Design review of the part built by this model. Coordinates are the model's own, in mm. A direction names the side the tool comes from. Coordinates: 2 decimals unless noted, no trailing zeros. Write item = value, one per line.
```python
from build123d import *

# Parameters (mm, degrees)
F1_DEPTH    = 9
F2_T        = -1.625
F3_R        = 4.65
F4_DEPTH    = 5.75
F6_DEPTH    = 9
F7_T4_DEPTH = 11.5292765407
F8_R        = 1.5
F9_R        = 1.5
F11_DEPTH   = 25
F12_R       = 1.65
F13_DEPTH   = 0.8125
F14_R       = 4.65
F14_R_2     = 1.65
F15_DEPTH   = 0.8125
F17_DEPTH   = 25
F19_DEPTH   = 25


# Not quite as in the source:
# - a fillet or chamfer that OpenCascade refuses, or shapes differently, is made with other operations: its cross-section is extruded or revolved along the edge and cut away or added


with BuildPart() as f1:
    # F0 (on Top) → F1 (new body)
    with BuildSketch(Plane.XY):
        with BuildLine():
            Line((-2.2380131875, 10.0346875), (0, 9.35))
            Line((0, 9.35), (9.2696152423, -6.7054445662))
            Line((9.2696152423, -6.7054445662), (0, -6.7054445662))
            Line((0, -6.7054445662), (4.6188021535, -14.7054445662))
            Line((4.6188021535, -14.7054445662), (12.7337168574, -14.7054445662))
            ThreePointArc((12.7337168574, -14.7054445662), (17.9298692801, -11.7054445662), (17.9298692801, -5.7054445662))
            Line((17.9298692801, -5.7054445662), (14, 1.101288694))
            ThreePointArc((14, 1.101288694), (12.0019915499, 16.2776695961), (21.3205080757, 28.4217967697))
            Line((21.3205080757, 28.4217967697), (25.6506350946, 30.9217967697))
            ThreePointArc((25.6506350946, 30.9217967697), (29.1558482852, 35.7019755006), (28, 41.5158075373))
            Line((28, 41.5158075373), (-6.2733497352, 21.7280798417))
            ThreePointArc((-6.2733497352, 21.7280798417), (-7.2315061235, 14.8544401058), (-2.2380131875, 10.0346875))
        make_face()
        with BuildLine():
            ThreePointArc((1.65, 17.35), (1.166726189, 16.183273811), (0, 15.7))
            ThreePointArc((0, 15.7), (-1.166726189, 18.516726189), (1.65, 17.35))
        make_face(mode=Mode.SUBTRACT)
    extrude(amount=F1_DEPTH)

    # F2
    f2_openings = [f1.faces().sort_by_distance(p)[0] for p in [
        (10.863325, 31.621944, 4.5),
        (-7.231506, 14.85444, 4.5),
        (4.634808, 1.322278, 4.5),
        (4.634808, -6.705445, 4.5),
        (2.309401, -10.705445, 4.5),
        (-1.119007, 9.692344, 4.5),
    ]]
    offset(amount=F2_T, openings=f2_openings)

    # F3 (on face) → F4 (cut, through all)
    with BuildSketch(Plane.XY.offset(1.625)):
        with Locations((0, 17.35)):
            Circle(F3_R)
    extrude(amount=F4_DEPTH, mode=Mode.SUBTRACT)

    # F5 (on face) → F6 (join)
    with BuildSketch(Plane.XY):
        Polygon((0, -6.7054445662), (4.6188021535, -14.7054445662), (6.9282032303, -14.7054445662), (2.3094010768, -6.7054445662), align=None)
    extrude(amount=F6_DEPTH)

    # F7: fillet of radius 2 on 2 edges, made by hand


with BuildPart() as f7_tool2:
    # F7_s3 → F7_t4 (new body)
    with BuildSketch(Plane.XY.offset(-1.2646382703)):
        with BuildLine():
            ThreePointArc((5.4117350132, -12.0796445662), (6.1446642818, -12.8125738348), (7.1458642818, -13.0808445662))
            Line((7.1458642818, -13.0808445662), (7.1458642818, -13.2810845662))
            ThreePointArc((7.1458642818, -13.2810845662), (6.5679366623, -13.2806845662), (5.9900090428, -13.2806845662))
            Line((5.9900090428, -13.2806845662), (5.816596116, -13.1805645662))
            ThreePointArc((5.816596116, -13.1805645662), (5.5276323063, -12.6800645662), (5.2383220864, -12.1797645662))
            Line((5.2383220864, -12.1797645662), (5.4117350132, -12.0796445662))
        make_face()
    extrude(amount=F7_T4_DEPTH)

    split(bisect_by=Plane.XY.offset(9), keep=Keep.BOTTOM)

    split(bisect_by=Plane.XY, keep=Keep.TOP)


with BuildPart() as f1_1:
    add(f1.part)

    # F7_t1: union F7_tool2
    add(f7_tool2.part)

    # F8
    f8_edges = [f1_1.edges().sort_by_distance(p)[0] for p in [
        (14.557643, -3.114578, 7.375),
    ]]
    fillet(f8_edges, radius=F8_R)

    # F9
    f9_edges = [f1_1.edges().sort_by_distance(p)[0] for p in [
        (10.432362, 16.698251, 1.625),
        (3.870747, -9.409775, 1.625),
        (27.584345, 36.123263, 1.625),
        (22.673072, 31.079088, 1.625),
        (14.557643, -3.114578, 1.625),
        (16.522578, -10.892945, 1.625),
        (9.91978, -13.080445, 1.625),
        (6.144664, -12.812574, 1.625),
    ]]
    fillet(f9_edges, radius=F9_R)

    # F10 (on face) → F11 (cut)
    with BuildSketch(Plane(origin=(0, 0, 0), x_dir=(1, 0, 0), z_dir=(0, 0, -1))):
        with BuildLine():
            ThreePointArc((0, -22), (-4.65, -17.35), (0, -12.7))
            Line((0, -12.7), (0, -9.35))
            Line((0, -9.35), (-2.2380131875, -10.0346875))
            ThreePointArc((-2.2380131875, -10.0346875), (-7.2315061235, -14.8544401058), (-6.2733497352, -21.7280798417))
            Line((-6.2733497352, -21.7280798417), (0, -25.35))
            Line((0, -25.35), (0, -22))
        make_face()
    extrude(amount=-F11_DEPTH, mode=Mode.SUBTRACT)

    # F12 (on face) → F13 (cut)
    with BuildSketch(Plane(origin=(0, 0, 0), x_dir=(1, 0, 0), z_dir=(0, 0, -1))):
        with BuildLine():
            ThreePointArc((0, -22), (3.2880465325, -20.6380465325), (4.65, -17.35))
            ThreePointArc((4.65, -17.35), (3.2880465325, -14.0619534675), (0, -12.7))
            ThreePointArc((0, -12.7), (-4.65, -17.35), (0, -22))
        make_face()
        with Locations((0, -17.35)):
            Circle(F12_R, mode=Mode.SUBTRACT)
        with Locations((0, -17.35)):
            Circle(F12_R)
    extrude(amount=-F13_DEPTH, mode=Mode.SUBTRACT)

    # F14 (on face) → F15 (cut)
    with BuildSketch(Plane(origin=(0, 0, 7.375), x_dir=(1, 0, 0), z_dir=(0, 0, -1))):
        with Locations((0, -17.35)):
            Circle(F14_R)
        with Locations((0, -17.35)):
            Circle(F14_R_2, mode=Mode.SUBTRACT)
    extrude(amount=-F15_DEPTH, mode=Mode.SUBTRACT)

    # F16 (on face) → F17 (cut)
    with BuildSketch(Plane(origin=(0, 0, 0), x_dir=(1, 0, 0), z_dir=(0, 0, -1))):
        with BuildLine():
            Line((6.9282032303, -29.35), (2.325, -21.3770181276))
            ThreePointArc((2.325, -21.3770181276), (1.2035085597, -21.8415550922), (0, -22))
            Line((0, -22), (0, -25.35))
            Line((0, -25.35), (6.9282032303, -29.35))
        make_face()
    extrude(amount=-F17_DEPTH, mode=Mode.SUBTRACT)

    # F18 (on face) → F19 (cut)
    with BuildSketch(Plane.XY.offset(9)):
        with BuildLine():
            Line((2.175, 21.1172105065), (2.325, 21.3770181276))
            ThreePointArc((2.325, 21.3770181276), (-4.4915550922, 18.5535085597), (0, 12.7))
            Line((0, 12.7), (0, 13))
            ThreePointArc((0, 13), (-4.2017773444, 18.4758628462), (2.175, 21.1172105065))
        make_face()
    extrude(amount=-F19_DEPTH, mode=Mode.SUBTRACT)


solid = f1_1.part
```
(1) For faces 1 (the cylindrical face through (27.57, 36.06, 4.48)), 2 (the flat face through (3.893, -9.448, 4.481)), 3 (the flat face through (4.57, 1.435, 8.176)), 4 (the flat face through (0, 11, 1)), 5 (the flat face through (10, -13.08, 4)), list the 3-axis set-ups (+Z, -Z, +X, -X, +Y, -Y) from which the entire face can be reached by the end or side of a thin tool; tool diameter is ignored.
Report:
face_1 = -X
face_2 = +Y
face_3 = +Z, -Z, -X
face_4 = +Z, -Z, -X, -Y
face_5 = none
(2) Insertion check: pin 1 (1.8 mm diameter, centred on y = 10.5, z = 8, fed in from -X); pin 2 (2.5 mm diameter, centred on x = 0.5, y = 18.5, fed in from -Z); pin 3 (1.5 mm diameter, centred on x = 14.5, z = 5, fed in from -Y). Each pin has a flat end and moves straight along its axis. Give the tip position at first contact, or say it passes through.
Report:
pin_1 = 0
pin_2 = 0.81
pin_3 = -14.62
(3) The part is to be moulded in two halves that separate along Z. For faces 6 (the cylindrical face through (9.88, -12.629, 6.947)), 7 (the flat face through (2, 17, 0.812)), 8 (the cylindrical face through (9.959, -12.629, 2.053)), 9 (the flat face through (15.992, -2.35, 4.437)), say which applies: released by +Z, released by -Z, zero draft, split by the parting line, or undercut.
Report:
face_6 = undercut
face_7 = released by -Z
face_8 = undercut
face_9 = zero draft
(4) We need section A-A (x = 3). Give the number of separate pieces and of enclosed holes in the cut face, and give its area (3 significant figures).
Report:
separate_pieces = 3
enclosed_holes = 0
area = 89.7 mm²
(5) For L1, parallel to Y at x = 14.5, z = 3.5; L2, parallel to Z at x = 4, y = 22 (3 decimals); L3, parallel to Y at x = 15.5, z = 6, list the stretches that pass through material, from the lowest coordinate up.
Report:
L1 = -14.44 to -12.71, -3.01 to 0.24, 21.92 to 24.69
L2 = 0 to 1.625, 7.375 to 9
L3 = -14.03 to -12.09, -4.76 to -1.5, 23.34 to 25.85
